Design review of the part shown in the three views and the two pictorial views. Dimensions are in mm from the part's minimum x, y and z. Give positions to 0.01 mm unless a question says otherwise; leave off trailing zeros. Loops run counter-clockwise (first coordinate to the right, second up) from the corner with the lowest first, then second, coordinate; pieces in that order, holes last. Notation, with made-up numbers: (14, -35.75) -> (23, -35.75) arc R9 ccw to (23, -27.75) -> close; hole circle Ø6 at (55.5, 77.25). An arc over 180 degrees is marked (long way). Answer as CSV lines item,"result". Start each with the question number.
Item 1: The part is to be moulded in two halves that separate along Y. For the marked faces 1, 2 and 3, say which applies: +Y half, -Y half, draft (parallel to the pull), parting line (faces both ways), or undercut.
Item 2: For L1, parallel to X at y = 283.5, z = 713, list the stretches that pass through material, from the lowest coordinate up. Write a range as from..to.
Item 3: Add section B-B on y = 545. State the section outline as (x, z) points.
Item 4: Add section A-A on z = 104.5. State the section outline as (x, y) points.
Item 5: Clearance check with a flat-ended pin moving along its axis: P1, Ø2, axis at y = 960, z = 241.5, coming from the -X side. State where the tip first meets the part, or that it passes through.
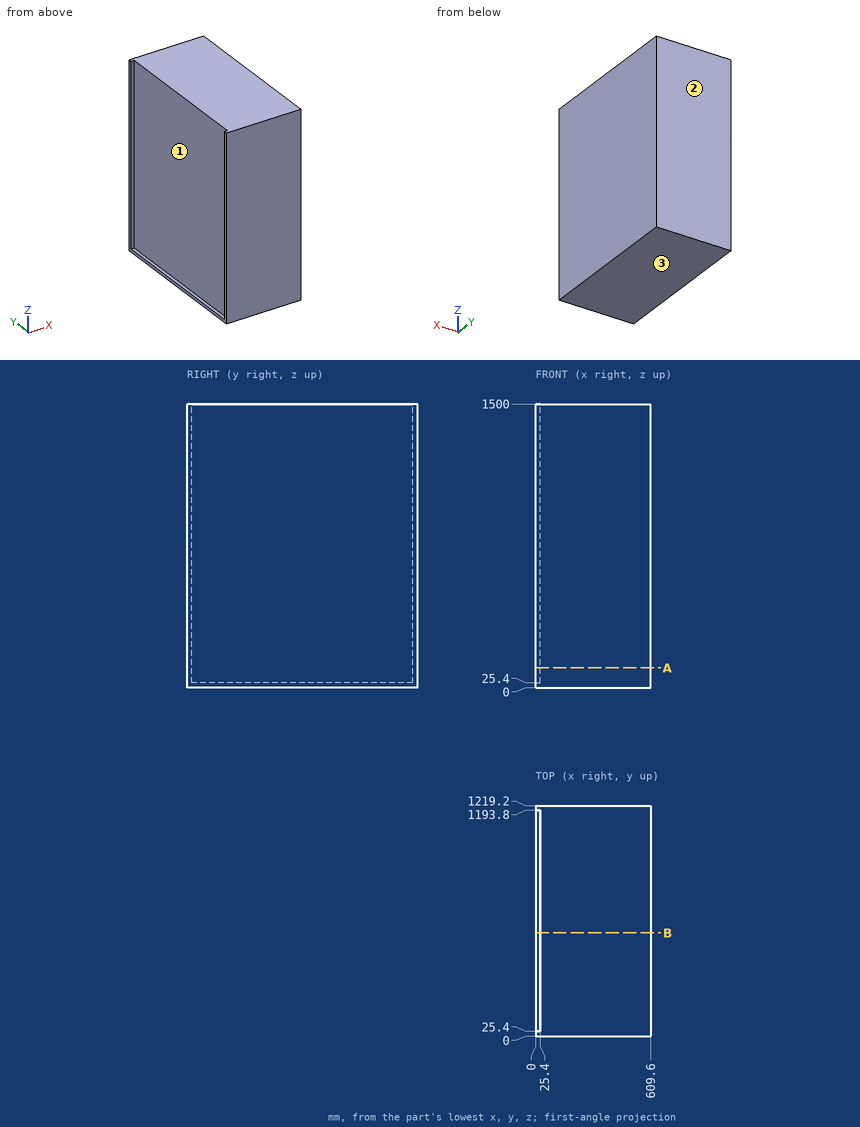
Computed values:
1,face 1,"undercut"
1,face 2,"+Y half"
1,face 3,"draft"
2,L1,"25.4..609.6"
3,outline,"(0, 0) -> (609.6, 0) -> (609.6, 1500) -> (25.4, 1500) -> (25.4, 25.4) -> (0, 25.4) -> close"
4,outline,"(0, 0) -> (609.6, 0) -> (609.6, 1219.2) -> (0, 1219.2) -> (0, 1193.8) -> (25.4, 1193.8) -> (25.4, 25.4) -> (0, 25.4) -> close"
5,P1,"x = 25.4"
